from build123d import *

# Parameters (mm, degrees)
EXTRUDE1_DEPTH      = 50.8
SKETCH2_R           = 4.0005
SKETCH2_R_2         = 1.1938
CUT_EXTRUDE1_DEPTH  = 27.9875
SKETCH22_R          = 4.0005
SKETCH22_R_2        = 1.1938
CUT_EXTRUDE12_DEPTH = 27.9875
LPATTERN1_COUNT     = 2
LPATTERN1_PITCH     = 25.4
FILLET1_R           = 2.286
FILLET2_R           = 3.175


with BuildPart() as part:
    # Sketch1 → Extrude1 (new body)
    with BuildSketch(Plane.XY):
        Polygon((11.20775, -26.9875), (11.20775, -2.286), (-11.20775, -2.286), (-11.20775, -26.9875), (-13.49375, -26.9875), (-13.49375, 0), (13.49375, 0), (13.49375, -26.9875), align=None)
    extrude(amount=-EXTRUDE1_DEPTH)

    # Sketch2 → Cut-Extrude1 (cut, through all)
    with BuildSketch(Plane(origin=(13.49375, -15.292465387, -16.409839131), x_dir=(0, 0, -1), z_dir=(1, 0, 0))):
        with Locations((-3.709839131, 1.792365387)):
            Circle(SKETCH2_R)
        with Locations((-3.709839131, 10.123565387)):
            Circle(SKETCH2_R_2)
        with Locations((4.621360869, 1.792365387)):
            Circle(SKETCH2_R_2)
        with Locations((-3.709839131, -6.538834613)):
            Circle(SKETCH2_R_2)
        with Locations((-12.041039131, 1.792365387)):
            Circle(SKETCH2_R_2)
    cut_extrude1 = extrude(amount=-CUT_EXTRUDE1_DEPTH, mode=Mode.SUBTRACT)

    # Sketch22 → Cut-Extrude12 (cut, through all)
    with BuildSketch(Plane(origin=(-3.640346977, 0, -15.26070859), x_dir=(-1, 0, 0), z_dir=(0, 1, 0))):
        with Locations(Location((-3.640346977, 2.56070859, 0), (0, 0, 90))):  # turned: the seam where the file's is
            Circle(SKETCH22_R)
        with Locations(Location((-3.640346977, 10.89190859, 0), (0, 0, 90))):  # turned: the seam where the file's is
            Circle(SKETCH22_R_2)
        with Locations(Location((4.690853023, 2.56070859, 0), (0, 0, 90))):  # turned: the seam where the file's is
            Circle(SKETCH22_R_2)
        with Locations(Location((-3.640346977, -5.77049141, 0), (0, 0, 90))):  # turned: the seam where the file's is
            Circle(SKETCH22_R_2)
        with Locations(Location((-11.971546977, 2.56070859, 0), (0, 0, 90))):  # turned: the seam where the file's is
            Circle(SKETCH22_R_2)
    cut_extrude12 = extrude(amount=-CUT_EXTRUDE12_DEPTH, mode=Mode.SUBTRACT)

    # LPattern1: Cut-Extrude1, Cut-Extrude12 ×2
    with Locations(*[(0, 0, -i * LPATTERN1_PITCH) for i in range(1, LPATTERN1_COUNT)]):
        add(cut_extrude1, mode=Mode.SUBTRACT)
        add(cut_extrude12, mode=Mode.SUBTRACT)

    # Fillet1
    fillet1_edges = [part.edges().sort_by_distance(p)[0] for p in [
        (-13.49375, 0, -25.4),
        (13.49375, 0, -25.4),
    ]]
    fillet(fillet1_edges, radius=FILLET1_R)

    # Fillet2
    fillet2_edges = [part.edges().sort_by_distance(p)[0] for p in [
        (12.35075, -26.9875, -50.8),
        (-12.35075, -26.9875, -50.8),
        (12.35075, -26.9875, 0),
        (-12.35075, -26.9875, 0),
    ]]
    fillet(fillet2_edges, radius=FILLET2_R)


solid = part.part
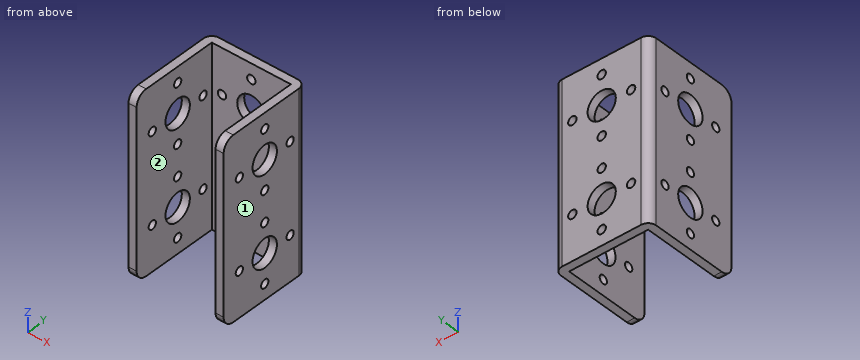
The model under review builds one solid part; all positions refer to its coordinate system, in mm. Face numbers are marked on the shaded views. A direction names the side the tool comes from. Give positions to 0.01 mm unless a question says otherwise; leave off trailing zeros. Order: outer loops, then holes, each group sorted by start corner. A loop starts at its lowest first (then second) coordinate and runs counter-clockwise, first axis right, second up. Notation, with made-up numbers: M 40.25,15 L 72.25,15 A25 ccw 72.25,52 Z; hole C 26,-2.5 d9. An arc over 180 degrees is marked long. Use one line per item in the form item = value. Start each with the question number.
Item 1: We need section B-B on z = -40. Give the boundary of the cut face in (x, y).
Item 2: We need section C-C on y = -3. Give the boundary of the cut face in (x, z).
Item 3: We need section A-A on x = 0. Give the boundary of the cut face in (y, z) (1 decimal), plus the area to 3 significant figures.
Item 4: We need section D-D on z = -7.5. Give the boundary of the cut face in (x, y), plus the area to 3 significant figures.
Item 5: To check wall thickness, follow line 1 along X through (y, z) = (-8, -10); line 2 along Z through (x, y) = (-12.5, -15); line 3 along Y through (x, z) = (-11.5, -12). State the ranges of each line that lie inside material, in increasing order. Write a range as from..to.
Item 6: Insertion check: pin 1 Ø7 at (y, z) = (-13.5, -12.7) entering from -X; pin 2 Ø11 at (x, z) = (-2, -36.5) entering from -Y. Each pin has a flat end and moves straight along its axis. Give the tip position at first contact, or say it passes through.
Item 7: For the marked faces 1 and 2, list the 3-axis set-ups (+Z, -Z, +X, -X, +Y, -Y) from which the entire face can be reached by the end or side of a thin tool; tool diameter is ignored.
Completed:
q1.outline = M -13.49,-26.99 L -11.21,-26.99 L -11.21,-17.02 L -13.49,-17.02 Z; M -13.49,-9.98 L -11.21,-9.98 L -11.21,-2.29 L -3.52,-2.29 L -3.52,0 L -11.21,0 A2.29 ccw -13.49,-2.29 Z; M 3.52,-2.29 L 11.21,-2.29 L 11.21,-9.98 L 13.49,-9.98 L 13.49,-2.29 A2.29 ccw 11.21,0 L 3.52,0 Z; M 11.21,-26.99 L 13.49,-26.99 L 13.49,-17.02 L 11.21,-17.02 Z
q2.outline = M -13.49,-50.8 L -11.21,-50.8 L -11.21,0 L -13.49,0 Z; M 11.21,-50.8 L 13.49,-50.8 L 13.49,0 L 11.21,0 Z
q3.outline = M -2.3,-50.8 L 0,-50.8 L 0,-47.6 L -2.3,-47.6 Z; M -2.3,-45.2 L 0,-45.2 L 0,-42.1 L -2.3,-42.1 Z; M -2.3,-34.1 L 0,-34.1 L 0,-31 L -2.3,-31 Z; M -2.3,-28.6 L 0,-28.6 L 0,-22.2 L -2.3,-22.2 Z; M -2.3,-19.8 L 0,-19.8 L 0,-16.7 L -2.3,-16.7 Z; M -2.3,-8.7 L 0,-8.7 L 0,-5.6 L -2.3,-5.6 Z; M -2.3,-3.2 L 0,-3.2 L 0,0 L -2.3,0 Z
q3.area = 57.7 mm²
q4.outline = M -13.49,-26.99 L -11.21,-26.99 L -11.21,-2.29 L 11.21,-2.29 L 11.21,-26.99 L 13.49,-26.99 L 13.49,-2.29 A2.29 ccw 11.21,0 L -11.21,0 A2.29 ccw -13.49,-2.29 Z
q4.area = 172 mm²
q5.line_1 = -13.49..-11.21, 11.21..13.49
q5.line_2 = -50.8..-41.81, -34.39..-16.41, -8.99..0
q5.line_3 = -26.99..-22.8, -20.86..-17.44, -9.56..-6.14, -4.2..-0.02
q6.pin_1 = through
q6.pin_2 = -2.29
q7.face_1 = +Z, -Z, +X, +Y, -Y
q7.face_2 = +Z, -Z, -Y
